The listing builds one solid part. Answer for the finished solid, in the listing's coordinates (mm). Face numbers are marked on the shaded views. Give positions to 0.01 mm unless a question says otherwise; leave off trailing zeros. Write each loop counter-clockwise with the first axis right and the second up, starting at its lowest first coordinate (ties: lowest second). Pieces come first, ordered by that corner, then holes.
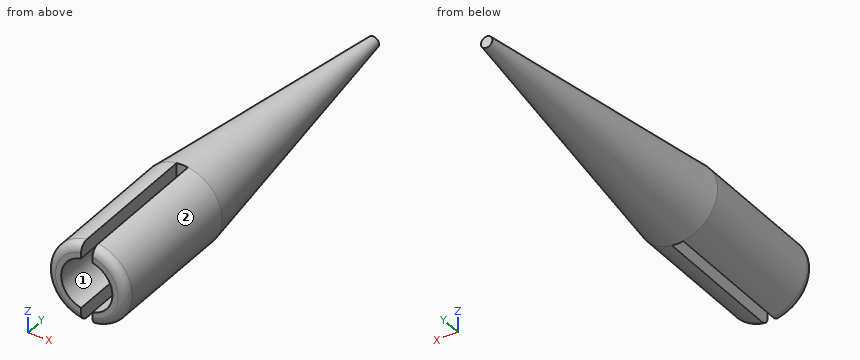
```python
from build123d import *

# Parameters (mm, degrees)
F0_R      = 7
F1_DEPTH  = 25
F3_R      = 1
F1_FACE_R = 7
F5_T      = -2.5
F6_R      = 1.5
F8_W      = 2
F8_H      = 21.4920276658
F9_DEPTH  = 25


# Not quite as in the source:
# - a shell that OpenCascade refuses in one call is made with other operations: the cavity is built on its own and cut out
# - a feature names something its author has since deleted; it is built from what else it names


with BuildPart() as f1:
    # F0 (on Front) → F1 (new body)
    with BuildSketch(Plane.XZ):
        Circle(F0_R)
    extrude(amount=F1_DEPTH)

    # F3 (on offset) → F4 section 0
    with BuildSketch(Plane.XZ.offset(-50)):
        Circle(F3_R)
    # F1_face (on face) → F4 section 1
    with BuildSketch(Plane(origin=(0, 0, 0), x_dir=(1, 0, 0), z_dir=(0, 1, 0))):
        Circle(F1_FACE_R)
    loft()

    # F5: a shell. OpenCascade refuses it in one call, so the cavity is built on its own and cut out:
    # the body offset inwards by the wall thickness, plus a prism from it out through each open face.
    f5_core = offset(f1.part, amount=F5_T, mode=Mode.PRIVATE)
    f5_exits = [f5_core.faces().sort_by_distance(p)[0] for p in [
        (0, -22.5, 0),
    ]]
    add(f5_core, mode=Mode.SUBTRACT)
    extrude(f5_exits, amount=-F5_T, mode=Mode.SUBTRACT)

    # F6
    f6_edges = [f1.edges().sort_by_distance(p)[0] for p in [
        (-7, -25, 0),
    ]]
    fillet(f6_edges, radius=F6_R)

    # F8 (on offset) → F9 (cut)
    with BuildSketch(Plane.XZ.offset(25)):
        Rectangle(F8_W, F8_H)
    extrude(amount=-F9_DEPTH, mode=Mode.SUBTRACT)


solid = f1.part
```
Item 1: A cutting plane is placed at A-A, the plane y = -9.5. Give the vertices of the cut face in (x, z), plus the area to 3 significant figures.
Conclusion:
outline: (-1, -6.93) - (-1, -4.39) arc R4.5 cw to (-1, 4.39) - (-1, 6.93) arc R7 ccw to start; (1, -6.93) arc R7 ccw to (1, 6.93) - (1, 4.39) arc R4.5 cw to (1, -4.39) - close
area: 80.3 mm2
Item 2: Consider probe 1 along X at (y, z) = (-7, -1); probe 2 along X at (y, z) = (-14, -0.5); probe 3 along Z at (x, y) = (0.75, 4). Determine where each line is inside the solid, lowest interval first.
Conclusion:
probe 1: x = -6.93 to -4.39, 4.39 to 6.93
probe 2: x = -6.98 to -4.47, 4.47 to 6.98
probe 3: z = -6.48 to -3.93, 3.93 to 6.48
Item 3: Determine the mould class of the marked faces 1 and 2 for opening direction Z: pulls with the +Z half, pulls with the -Z half, needs draft (parallel to the pull), parting line crosses it, or undercut.
Conclusion:
face 1: undercut
face 2: parting line crosses it
Item 4: Each of these flat-tipped pins is pushed along its axis until it touches: P1, Ø3, axis at x = 2, y = -9, coming from the +Z side; P2, Ø1.6, axis at x = 0, z = 6, coming from the -Y side; P3, Ø0.8, axis at y = -9, z = 6, coming from the +X side. Where does it stop, or does it pass through?
Conclusion:
P1: stops at z = 6.93
P2: stops at y = 0
P3: stops at x = 4.2
